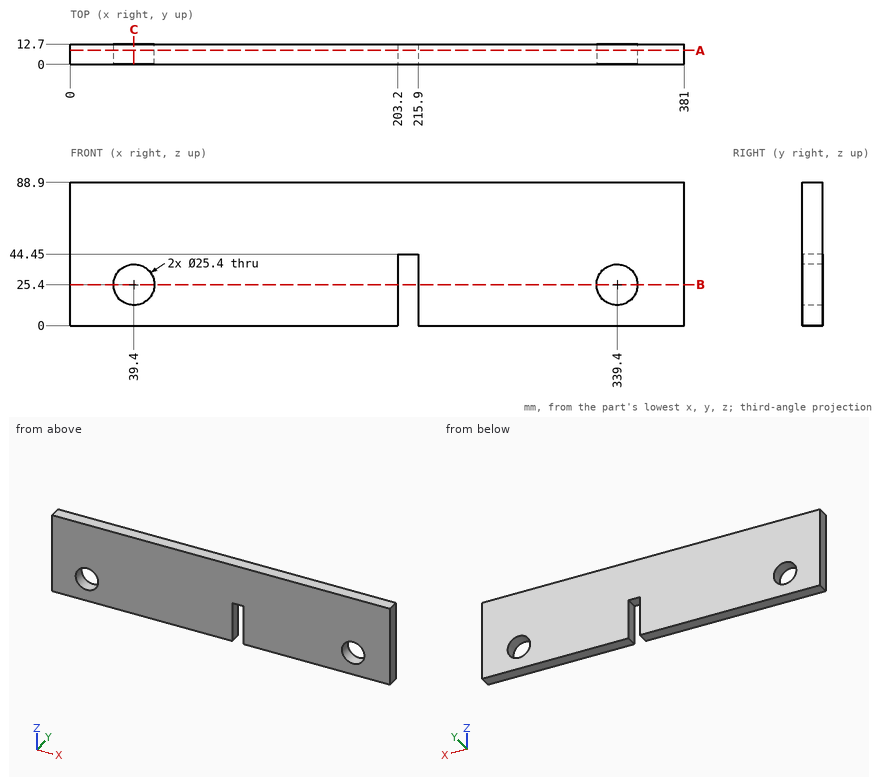
Study the drawing (mm; zero at the part's minimum x, y, z) and answer. Round coordinates to 2 decimals unless told otherwise and drop trailing zeros. Order: outer loops, then holes, each group sorted by start corner. A loop starts at its lowest first (then second) coordinate and runs counter-clockwise, first axis right, second up. Notation, with made-up numbers: (88.5, 52.25) - (117.5, 52.25) arc R24 cw to (117.5, 87.25) - close; hole circle Ø8 at (27.25, 80.25). An arc over 180 degrees is marked (long way). Use one line per item in the form item = value. Start each with the question number.
(1) The part is cut by section A-A (y = 8.75). Give the vertices of the cut face in (x, z), then the cut area to 3 significant figures.
(2) Find the intervals of material crossed by line 1 along X through (y, z) = (6.75, 25.5); line 2 along X through (y, z) = (8, 21); line 3 along Z through (x, y) = (339.4, 5.75), in increasing order. Write a range as from..to.
(3) The part is cut by section B-B (z = 25.4). Give the vertices of the cut face in (x, y), then the cut area to 3 significant figures.
(4) The part is cut by section C-C (x = 39.4). Give the vertices of the cut face in (y, z), then the cut area to 3 significant figures.
(5) A flat-ended cylindrical pin translates along its axis: pin 1 Ø20.5 at (x, z) = (39.4, 25.4) entering from -Y. Find the tip coordinate at first contact, or state that the pin passes through.
Checked values:
q1.outline = (0, 0) - (203.2, 0) - (203.2, 44.45) - (215.9, 44.45) - (215.9, 0) - (381, 0) - (381, 88.9) - (0, 88.9) - close; hole circle Ø25.4 at (39.4, 25.4); hole circle Ø25.4 at (339.4, 25.4)
q1.area = 32,300 mm^2
q2.line_1 = 0..26.7, 52.1..203.2, 215.9..326.7, 352.1..381
q2.line_2 = 0..27.49, 51.31..203.2, 215.9..327.49, 351.31..381
q2.line_3 = 0..12.7, 38.1..88.9
q3.outline = (0, 0) - (26.7, 0) - (26.7, 12.7) - (0, 12.7) - close; (52.1, 0) - (203.2, 0) - (203.2, 12.7) - (52.1, 12.7) - close; (215.9, 0) - (326.7, 0) - (326.7, 12.7) - (215.9, 12.7) - close; (352.1, 0) - (381, 0) - (381, 12.7) - (352.1, 12.7) - close
q3.area = 4,030 mm^2
q4.outline = (0, 0) - (12.7, 0) - (12.7, 12.7) - (0, 12.7) - close; (0, 38.1) - (12.7, 38.1) - (12.7, 88.9) - (0, 88.9) - close
q4.area = 806 mm^2
q5.pin_1 = through
